```python
from build123d import *

# Parameters (mm, degrees)
F0_R     = 25.4
F1_DEPTH = 6.35
F2_R     = 3.96875
F3_DEPTH = 25.4
F2_R_2   = 25.4
F2_R_3   = 22.225
F4_DEPTH = 6.35
F5_SIZE  = 2.54


with BuildPart() as f1:
    # F0 (on Top) → F1 (new body)
    with BuildSketch(Plane.XY):
        Circle(F0_R)
    extrude(amount=F1_DEPTH)

    # F2 (on face) → F3 (cut)
    with BuildSketch(Plane(origin=(0, 0, 0), x_dir=(1, 0, 0), z_dir=(0, 0, -1))):
        Circle(F2_R)
    extrude(amount=-F3_DEPTH, mode=Mode.SUBTRACT)

    # F2 (on face) → F4 (join)
    with BuildSketch(Plane(origin=(0, 0, 0), x_dir=(1, 0, 0), z_dir=(0, 0, -1))):
        Circle(F2_R_2)
        Circle(F2_R_3, mode=Mode.SUBTRACT)
    extrude(amount=F4_DEPTH)

    # F5
    f5_edges = [f1.edges().sort_by_distance(p)[0] for p in [
        (-3.96875, 0, 6.35),
        (-25.4, 0, 6.35),
    ]]
    chamfer(f5_edges, length=F5_SIZE)


solid = f1.part
```
Design review of the part built by this model. Coordinates are the model's own, in mm. A direction names the side the tool comes from. Give positions to 0.01 mm unless a question says otherwise; leave off trailing zeros. Order: outer loops, then holes, each group sorted by start corner. A loop starts at its lowest first (then second) coordinate and runs counter-clockwise, first axis right, second up. Notation, with made-up numbers: (36.25, 44) - (90.25, 44) arc R24 ccw to (90.25, 61) - close; hole circle Ø6 at (-38.5, 13.5). An arc over 180 degrees is marked (long way). Use a Markdown table: item, result. Add a question column.
(1) Add section C-C on z = -2.5. Give the boundary of the cut face in (x, y) (3 decimals), then the cut area to 3 significant figures.
(2) Add section D-D on z = 1.25. Give the boundary of the cut face in (x, y), then the cut area to 3 significant figures.
(3) Clearance check with flat-ended pins moving along their axes: P1, Ø6, axis at x = 0.5, z = 0, coming from the -Y side; P2, Ø6, axis at y = -6.5, z = 3.5, coming from the -X side; P3, Ø1, axis at x = 12.5, y = 15.5, coming from the -Z side. State where each tip first meets the part, or that it passes through.
(4) Mouldability with a two-part tool opening along Y and no side actions: class faces 3 (the face through (-0.1, 22.5, -6.35)), 4 (the face through (0, -5, 0)), 5 (the face through (-5.506, 24.796, -1.199)), 6 (the face through (-0.89, 3.99, 3.93)) as +Y half, -Y half, draft (parallel to the pull), parting line (faces both ways), or undercut.
(5) Add section A-A on y = 0. Give the boundary of the cut face in (x, z) (3 decimals), then the cut area to 3 significant figures.
(6) Machinability: for faces 1 (the face through (-0.86, 3.874, 1.878)), 2 (the face through (21.199, -6.676, -3.131)), which of the approach directions +Z, -Z, +X, -X, +Y, -Y give a long, thin tool a straight path to every point of the face, cutting with its end or side? Answer none if there is none.
(7) Wall thickness on probe 1 along X at (y, z) = (0, 2.05); probe 2 along X at (y, z) = (0, -3.25) (3 decimals): over which ranges is each line inside the solid? List them lowest first. Write a range as [from, to].
Report:
| question | item | result |
|---|---|---|
| 1 | outline | circle Ø50.8 at (0, 0); hole circle Ø44.45 at (0, 0) |
| 1 | area | 475 mm² |
| 2 | outline | circle Ø50.8 at (0, 0); hole circle Ø7.94 at (0, 0) |
| 2 | area | 1,980 mm² |
| 3 | P1 | stops at y = -25.4 |
| 3 | P2 | stops at x = -25.16 |
| 3 | P3 | stops at z = 0 |
| 4 | face 3 | draft |
| 4 | face 4 | undercut |
| 4 | face 5 | parting line |
| 4 | face 6 | undercut |
| 5 | outline | (-25.4, -6.35) - (-22.225, -6.35) - (-22.225, 0) - (-3.969, 0) - (-3.969, 3.81) - (-6.509, 6.35) - (-22.86, 6.35) - (-25.4, 3.81) - close; (3.969, 0) - (22.225, 0) - (22.225, -6.35) - (25.4, -6.35) - (25.4, 3.81) - (22.86, 6.35) - (6.509, 6.35) - (3.969, 3.81) - close |
| 5 | area | 300 mm² |
| 6 | face 1 | +Z, -Z |
| 6 | face 2 | -Z |
| 7 | probe 1 | x = [-25.4, -3.97], [3.97, 25.4] |
| 7 | probe 2 | x = [-25.4, -22.225], [22.225, 25.4] |
